Part print with two shaded views. Sizes in mm from the minimum x, y, z corner. A direction names the side the tool comes from. Coordinates: 2 decimals unless noted, no trailing zeros. Loops run counter-clockwise (first coordinate to the right, second up) from the corner with the lowest first, then second, coordinate; pieces in that order, holes last.
(1) Tool access for the marked faces 5, 6 and 7: list every direction of +Z, -Z, +X, -X, +Y, -Y with a clear straight run to the whole face (end or side of a thin tool).
(2) Wall check: L1, parallel to Z at x = 2.5, y = 10.5; L2, parallel to Y at x = 7.5, z = 6; L3, parallel to Z at x = 13.5, y = 11.5. Give the ranges that are in metal, low to high.
(3) Slice it at A-A (z = 10.25). Give the cut face in (x, y).
(4) Slice it at B-B (x = 1). Give the cut face in (y, z), and give its area (4 significant figures).
(5) Two-plate mould, pull along Z, no slides. Class the marked faces 1, 2, 3 and 4: pulls with the +Z half, pulls with the -Z half, needs draft (parallel to the pull), parting line crosses it, or undercut.
(6) Flat gauge pins, fed straight in: P1, Ø2, axis at y = 4.5, z = 6, coming from the +X side; P2, Ø2, axis at y = 8, z = 10, coming from the -X side; P3, Ø3.5, axis at x = 8.5, y = 10, coming from the +Z side. Where does each tip first touch, or does it go through?
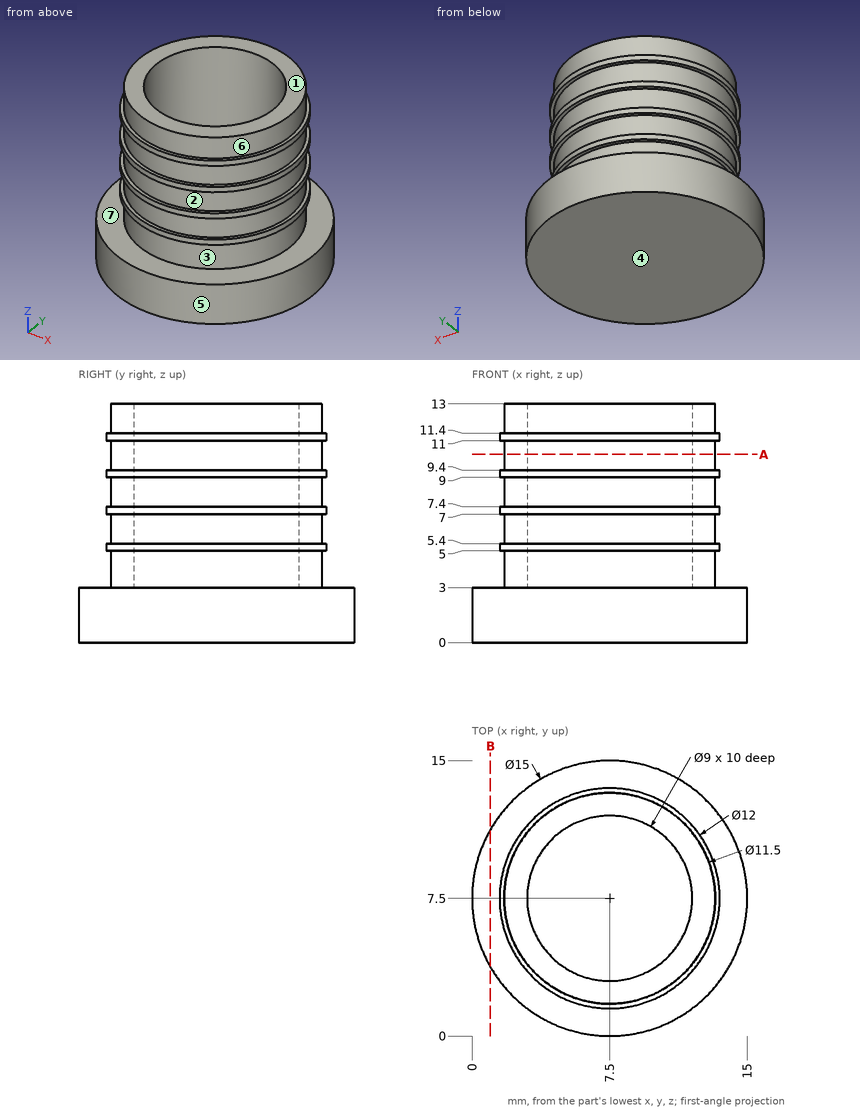
Response values:
1. face 5: +Z, -Z
1. face 6: +Z
1. face 7: none
2. L1: z = 0 to 3, 5 to 5.4, 7 to 7.4, 9 to 9.4, 11 to 11.4
2. L2: y = 1.75 to 3, 12 to 13.25
2. L3: z = 0 to 3
3. outline: circle Ø11.5 at (7.5, 7.5); hole circle Ø9 at (7.5, 7.5)
4. outline: (3.76, 0) - (11.24, 0) - (11.24, 3) - (3.76, 3) - close
4. area: 22.45 mm2
5. face 1: pulls with the +Z half
5. face 2: undercut
5. face 3: undercut
5. face 4: pulls with the -Z half
6. P1: stops at x = 13.08
6. P2: stops at x = 1.5
6. P3: stops at z = 3
